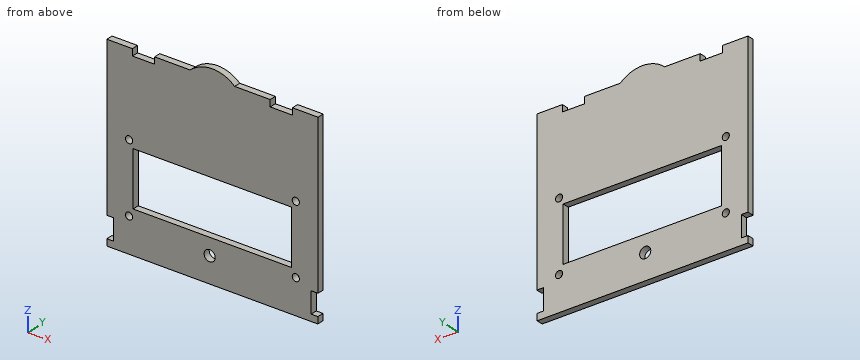
Autodesk Inventor part; units mm, degrees
ref_plane "YZ Plane" through (0, 0, 0) normal (1, 0, 0) x (0, 1, 0)
ref_plane "XZ Plane" through (0, 0, 0) normal (0, 1, 0) x (-1, 0, 0)
ref_plane "XY Plane" through (0, 0, 0) normal (0, 0, 1) x (1, 0, 0)
sketch "Esboço3" plane through (0, 0, 0) normal (0, 1, 0) x (-1, 0, 0)
  line L0 (0, 0) -> (-95, 0)
  line L1 (-95, 0) -> (-95, -80)
  line L2 (-95, -80) -> (0, -80)
  line L3 (0, -80) -> (0, 0)
  line L4 (-11.825, -65) -> (-83.175, -65)
  line L5 (-83.175, -65) -> (-83.175, -40.48)
  line L6 (-83.175, -40.48) -> (-11.825, -40.48)
  line L7 (-11.825, -40.48) -> (-11.825, -65)
  circle A0 centre (-46.25, -72.5) radius 2.5
  point P0 (-47.5, -40.48)
  dimension "d4" = 95
  dimension "d5" = 80
  dimension "d9" = 71.35
  dimension "d10" = 24.52
  dimension "d11" = 11.825
  dimension "d17" = 5
  dimension "d56" = 15
  dimension "d140" = 11.825
  dimension "d251" = 40.48
  dimension "d259" = 7.5
extrude "Extrusão2" add sketch "Esboço3" along normal blind 3
sketch "Esboço7" plane through (0, 3, 0) normal (0, 1, 0) x (1, 0, 0)
  line L0 (10, 68.48) -> (85, 68.48)
  line L1 (85, 68.48) -> (85, 37.48)
  line L2 (85, 37.48) -> (10, 37.48)
  line L3 (10, 37.48) -> (10, 68.48)
  line L4 (11.825, 40.48) -> (11.825, 65)
  line L5 (83.175, 65) -> (83.175, 40.48)
  line L6 (11.825, 65) -> (83.175, 65)
  line L7 (83.175, 40.48) -> (11.825, 40.48)
  circle A0 centre (10, 37.48) radius 1.6
  circle A1 centre (10, 68.48) radius 1.6
  circle A2 centre (85, 68.48) radius 1.6
  circle A3 centre (85, 37.48) radius 1.6
  point P0 (0, 0)
  dimension "d57" = 75
  dimension "d58" = 31
  dimension "d59" = 1.825
  dimension "d60" = 73.175
  dimension "d62" = 1.825
  dimension "d65" = 3.2
  dimension "d66" = 3.2
  dimension "d67" = 3.2
  dimension "d68" = 3.2
  dimension "d69" = 3
extrude "Extrusão4" cut sketch "Esboço7" against normal blind 3 contours L3 A1 L0 | L0 A1 L3 | A2 L1 L0 | L0 L1 A2 | A0 L2 L3 | L3 L2 A0 | A3 L2 L1 | L1 L2 A3
sketch "Esboço19" plane through (0, 3, 0) normal (0, 1, 0) x (1, 0, 0)
  line L0 (0, 0) -> (95, 0)
  arc A0 (37.5, 0) -> (57.5, 0) centre (47.5, 11.1803) ccw
  dimension "d189" = 20
  dimension "d190" = 15
  dimension "d191" = 37.5
extrude "Extrusão14" add sketch "Esboço19" against normal blind 3
sketch "Esboço23" plane through (0, 3, 0) normal (0, 1, 0) x (1, 0, 0)
  line L0 (0, 80) -> (0, 0)
  line L1 (0, 80) -> (95, 80)
  line L2 (95, 80) -> (95, 84)
  line L3 (95, 84) -> (0, 84)
  line L4 (0, 84) -> (0, 80)
  dimension "d208" = 4
extrude "Extrusão17" add sketch "Esboço23" against normal blind 3
sketch "Esboço24" plane through (0, 3, 0) normal (0, 1, 0) x (1, 0, 0)
  line L0 (95, 0) -> (95, 84)
  line L1 (95, 71.5) -> (91.9, 71.5)
  line L2 (91.9, 71.5) -> (91.9, 84)
  line L3 (91.9, 84) -> (95, 84)
  line L4 (95, 84) -> (95, 71.5)
  line L5 (95, 84) -> (0, 84)
  point P0 (0, 0)
  point P1 (93.45, 84)
  dimension "d211" = 3.1
  dimension "d212" = 12.5
  dimension "d213" = 0
extrude "Extrusão18" cut sketch "Esboço24" against normal blind 3
sketch "Esboço27" plane through (0, 3, 0) normal (0, 1, 0) x (1, 0, 0)
  line L0 (91.9, 84) -> (0, 84)
  line L1 (0, 84) -> (3, 84)
  line L2 (3, 84) -> (3, 71.5)
  line L3 (3, 71.5) -> (0, 71.5)
  line L4 (0, 71.5) -> (0, 84)
  point P0 (0, 0)
  dimension "d226" = 3
  dimension "d227" = 12.5
extrude "Extrusão21" cut sketch "Esboço27" against normal blind 3
sketch "Esboço29" plane through (0, 3, 0) normal (0, 1, 0) x (1, 0, 0)
  line L0 (57.5, 0) -> (95, 0)
  line L1 (83.5, 0) -> (73.5, 0)
  line L2 (73.5, 0) -> (73.5, 3)
  line L3 (73.5, 3) -> (83.5, 3)
  line L4 (83.5, 3) -> (83.5, 0)
  line L5 (21.5, 0) -> (11.5, 0)
  line L6 (11.5, 0) -> (11.5, 3)
  line L7 (11.5, 3) -> (21.5, 3)
  line L8 (21.5, 3) -> (21.5, 0)
  line L9 (0, 71.5) -> (0, 0)
  line L10 (95, 0) -> (95, 71.5)
  point P0 (11.5, 1.5)
  point P1 (83.5, 1.5)
  dimension "d241" = 10
  dimension "d242" = 3
  dimension "d243" = 10
  dimension "d244" = 3
  dimension "d245" = 11.5
  dimension "d246" = 11.5
extrude "Extrusão23" cut sketch "Esboço29" against normal blind 3
sketch "Esboço30" plane through (0, 3, 0) normal (0, 1, 0) x (1, 0, 0)
  line L0 (91.9, 71.5) -> (91.9, 84)
  line L1 (91.9, 84) -> (94.9, 84)
  line L2 (94.9, 84) -> (94.9, 81)
  line L3 (94.9, 81) -> (91.9, 81)
  line L4 (91.9, 81) -> (91.9, 84)
  line L5 (3, 71.5) -> (3, 84)
  line L6 (3, 84) -> (0, 84)
  line L7 (0, 84) -> (0, 81)
  line L8 (0, 81) -> (3, 81)
  line L9 (3, 81) -> (3, 84)
  point P0 (0, 0)
  dimension "d253" = 3
  dimension "d254" = 3
  dimension "d255" = 3
  dimension "d256" = 3
extrude "Extrusão24" add sketch "Esboço30" against normal blind 3
properties part number "Tampa"
Can you work these out from the model? Positions are in its coordinate system, mm. Coordinates: 2 decimals unless noted, no trailing zeros. Order: outer loops, then holes, each group sorted by start corner. A loop starts at its lowest first (then second) coordinate and runs counter-clockwise, first axis right, second up. Notation, with made-up numbers: (47, -3.5) - (84, -3.5) arc R18 cw to (84, 24.5) - close; hole circle Ø9 at (73.25, 88). An arc over 180 degrees is marked (long way). Answer as a JSON object with one key per item and string values. Group by question number.
Q1. Imagine slicing it at B-B (z = -56.5). Please give me the cut outline in (x, y) (3 decimals), and give its area (4 significant figures).
Q2. Will these pins go through, and if not, where does the flat tip stop? P1, Ø1.5, axis at x = 92, y = 2, coming from the +Z side; P2, Ø0.9, axis at x = 76.5, y = 1.5, coming from the +Z side.
Q3. I need wall thicknesses on line 1 (X direction, y = 1.85, z = -37.48); line 2 (Z direction, x = 85, y = 1.4); line 3 (Z direction, x = 22, y = 0.4). Which ranges of each line are inside material? Lowest first, please. Write a range as from..to.
Q4. Imagine slicing it at C-C (y = 2.3). Give the number of separate pieces and of enclosed holes in the cut face, and give its area (3 significant figures).
Q5. Imagine slicing it at A-A (x = 17). Please give me the cut outline in (y, z).
Q6. Imagine slicing it at D-D (x = 85). Please give me the cut outline in (y, z), and give its area (3 significant figures).
Determined:
{
 "1": {"outline": "(0, 0) - (11.825, 0) - (11.825, 3) - (0, 3) - close; (83.175, 0) - (95, 0) - (95, 3) - (83.175, 3) - close", "area": "70.95 mm2"},
 "2": {"P1": "stops at z = 0", "P2": "stops at z = -3"},
 "3": {"line 1": "x = 0..8.4, 11.6..83.4, 86.6..95", "line 2": "z = -84..-70.08, -66.88..-39.08, -35.88..0", "line 3": "z = -84..-65, -40.48..0"},
 "4": {"separate pieces": "1", "enclosed holes": "6", "area": "6,110 mm2"},
 "5": {"outline": "(0, -84) - (3, -84) - (3, -65) - (0, -65) - close; (0, -40.48) - (3, -40.48) - (3, -3) - (0, -3) - close"},
 "6": {"outline": "(0, -84) - (3, -84) - (3, -70.08) - (0, -70.08) - close; (0, -66.88) - (3, -66.88) - (3, -39.08) - (0, -39.08) - close; (0, -35.88) - (3, -35.88) - (3, 0) - (0, 0) - close", "area": "233 mm2"}
}
